Model file for the job. Use its own axes, mm. A direction names the side the tool comes from. Round coordinates to 2 decimals unless told otherwise and drop trailing zeros. Order: outer loops, then holes, each group sorted by start corner. A loop starts at its lowest first (then second) coordinate and runs counter-clockwise, first axis right, second up. Notation, with made-up numbers: (49.25, 50.5) -> (83.25, 50.5) arc R26 ccw to (83.25, 64.5) -> close; hole circle Ø8 at (12, 60.25). An arc over 180 degrees is marked (long way). Use CSV: the item, a comma, the result in double quotes.
```python
from build123d import *

# Parameters (mm, degrees)
SKETCH1_W           = 42.3
SKETCH1_H           = 42.3
BOSS_EXTRUDE1_DEPTH = 50
SKETCH2_R           = 11
BOSS_EXTRUDE2_DEPTH = 2
BOSS_EXTRUDE3_START = -2
SKETCH3_R           = 2.5
BOSS_EXTRUDE3_DEPTH = 24
SKETCH4_R           = 2
CUT_EXTRUDE1_DEPTH  = 4.5


with BuildPart() as part:
    # Sketch1 → Boss-Extrude1 (new body)
    with BuildSketch(Plane(origin=(0, 0, 0), x_dir=(0, 0, -1), z_dir=(1, 0, 0))):
        Rectangle(SKETCH1_W, SKETCH1_H)
    extrude(amount=BOSS_EXTRUDE1_DEPTH)

    # Sketch2 → Boss-Extrude2 (add)
    with BuildSketch(Plane(origin=(0, 0, 0), x_dir=(0, 0, -1), z_dir=(1, 0, 0))):
        Circle(SKETCH2_R)
    extrude(amount=-BOSS_EXTRUDE2_DEPTH)

    # Sketch3 → Boss-Extrude3 (add)
    with BuildSketch(Plane(origin=(0, 0, 0), x_dir=(0, 0, -1), z_dir=(1, 0, 0)).offset(BOSS_EXTRUDE3_START)):
        Circle(SKETCH3_R)
    extrude(amount=-BOSS_EXTRUDE3_DEPTH)

    # Sketch4 → Cut-Extrude1 (cut)
    with BuildSketch(Plane(origin=(0, 0, 0), x_dir=(0, 0, -1), z_dir=(1, 0, 0))):
        with Locations((15.5, 16.5)):
            Circle(SKETCH4_R)
        with Locations((15.5, -16.5)):
            Circle(SKETCH4_R)
        with Locations((-15.5, -16.5)):
            Circle(SKETCH4_R)
        with Locations((-15.5, 16.5)):
            Circle(SKETCH4_R)
    extrude(amount=CUT_EXTRUDE1_DEPTH, mode=Mode.SUBTRACT)


solid = part.part
```
Q1. Probe line 1 along Z through (x, y) = (2, -16); line 2 along Y through (x, z) = (2.5, -15.5); line 3 along Y through (x, z) = (1, 15). List the from-to ranges inside material, lowest first.
From the geometry:
line 1,"z = -21.15 to -17.44, -13.56 to 13.56, 17.44 to 21.15"
line 2,"y = -21.15 to -18.5, -14.5 to 14.5, 18.5 to 21.15"
line 3,"y = -21.15 to -18.44, -14.56 to 14.56, 18.44 to 21.15"
Q2. Which spindle directions (+Z, -Z, +X, -X, +Y, -Y) get a long thin tool onto all of the face, cutting with end or side? Do faces 5 (the cylindrical face through (2.218, -14.517, -15.24)), 6 (the flat face through (25, 0, 21.15)). Say none if no direction does.
From the geometry:
face 5,"-X"
face 6,"+Z, +X, -X, +Y, -Y"
Q3. Cut at A-A (z = -15.5). Give the cut face in (x, y).
From the geometry:
outline,"(0, -21.15) -> (50, -21.15) -> (50, 21.15) -> (0, 21.15) -> (0, 18.5) -> (4.5, 18.5) -> (4.5, 14.5) -> (0, 14.5) -> (0, -14.5) -> (4.5, -14.5) -> (4.5, -18.5) -> (0, -18.5) -> close"
Q4. Mould opens along Z. For faces 1 (the flat face through (-26, 0, 0)), 2 (the flat face through (4.5, -16, 16)), 3 (the cylindrical face through (-13.83, -2.44, 0.54)), 4 (the flat face through (25, 0, -21.15)) say: +Z half, -Z half, draft (parallel to the pull), parting line (faces both ways), or undercut.
From the geometry:
face 1,"draft"
face 2,"undercut"
face 3,"parting line"
face 4,"-Z half"
Q5. Pin check, flat tips, straight feed: pin 1 (1.5 mm diameter, centred on y = -7, z = 7, fed in from -X); pin 2 (1.2 mm diameter, centred on y = -17, z = -16.5, fed in from -X); pin 3 (2 mm diameter, centred on y = 17.5, z = -14.5, fed in from -X). Stop position of each tip, or through.
From the geometry:
pin 1,"stops at x = -2"
pin 2,"stops at x = 4.5"
pin 3,"stops at x = 0"
Q6. Cut at B-B (y = -16.5). Give the cut face in (x, z).
From the geometry:
outline,"(0, -21.15) -> (50, -21.15) -> (50, 21.15) -> (0, 21.15) -> (0, 17.5) -> (4.5, 17.5) -> (4.5, 13.5) -> (0, 13.5) -> (0, -13.5) -> (4.5, -13.5) -> (4.5, -17.5) -> (0, -17.5) -> close"
Q7. Cut at D-D (z = 6). Give the cut face in (x, y).
From the geometry:
outline,"(-2, -9.22) -> (0, -9.22) -> (0, -21.15) -> (50, -21.15) -> (50, 21.15) -> (0, 21.15) -> (0, 9.22) -> (-2, 9.22) -> close"
Q8. Cut at C-C (x = -7.5). Give the cut face in (y, z), plus the area to 3 significant figures.
From the geometry:
outline,"circle Ø5 at (0, 0)"
area,"19.6 mm²"
